Can you work these out from the model? Positions are in its coordinate system, mm. Face numbers are marked on the shaded views. A direction names the side the tool comes from. Coordinates: 2 decimals unless noted, no trailing zeros. Order: outer loops, then holes, each group sorted by start corner. A loop starts at its lowest first (then second) coordinate and runs counter-clockwise, first axis right, second up. Notation, with made-up numbers: M 15.25,40.5 L 38.25,40.5 A23 ccw 38.25,49.5 Z; hole C 70.5,29 d9. An arc over 180 degrees is marked long. Answer as CSV lines item,"result". Start each with the question number.
1. If we section it at A-A (x = 0): List the corners of the cut face in (y, z) for me.
2. If we mould it in two halves opening along Z, with no side actions, what happens to the marked faces 1, 2 and 3? For each: released by +Z, released by -Z, zero draft, split by the parting line, or undercut.
3. If we section it at C-C (z = -5): List the corners of the cut face in (x, y) for me.
4. If we section it at B-B (z = 0): List the corners of the cut face in (x, y) for me.
5. On a 3-axis mill with a long thin cutter (end or side, diameter ignored), from which of +Z, -Z, +X, -X, +Y, -Y can I reach the whole of each face in a straight line? I mean the marked faces 4, 5, 6 and 7. Say none if no direction works.
6. If we section it at D-D (x = 21): List the corners of the cut face in (y, z) for me, plus the area to 3 significant figures.
7. Will these pins go through, and if not, where does the flat tip stop? pin 1 (2 mm diameter, centred on y = 2.5, z = -11.5, fed in from +X); pin 2 (5 mm diameter, centred on y = 1, z = -11, fed in from -X); pin 3 (4.5 mm diameter, centred on x = -17, y = 4.5, fed in from +Z); pin 4 (2 mm diameter, centred on x = -21.92, z = 0, fed in from -Y).
8. I need wall thicknesses on line 1 along X through (y, z) = (7.9, 0); line 2 along X through (y, z) = (6, 0); line 3 along Z through (x, y) = (-22, 5). Which ranges of each line are inside material? Lowest first, please. Write a range as from..to.
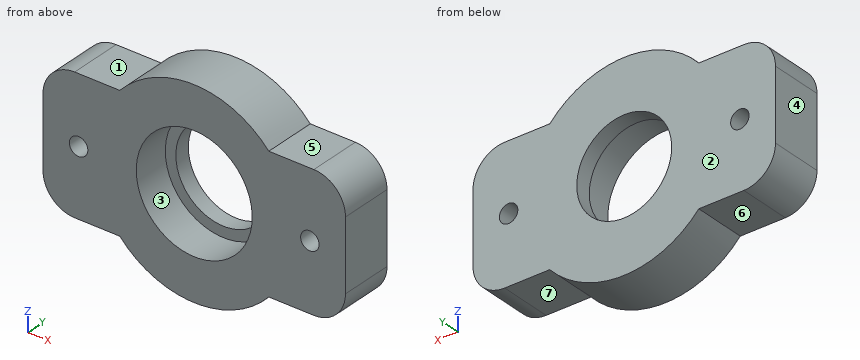
```python
from build123d import *

# Parameters (mm, degrees)
SKETCH1_R           = 11
SKETCH1_R_2         = 1.75
BOSS_EXTRUDE1_DEPTH = 10
BOSS_EXTRUDE2_START = -3
SKETCH2_R           = 11
SKETCH2_R_2         = 9
BOSS_EXTRUDE2_DEPTH = 3
FILLET1_R           = 6


with BuildPart() as part:
    # Sketch1 → Boss-Extrude1 (new body)
    with BuildSketch(Plane(origin=(0, 0, 0), x_dir=(1, 0, 0), z_dir=(0, 1, 0))):
        with BuildLine():
            Line((28.670310217, -12.7), (14.131878856, -12.7))
            ThreePointArc((14.131878856, -12.7), (0, -19), (-14.131878856, -12.7))
            Line((-14.131878856, -12.7), (-28.670310217, -12.7))
            Line((-28.670310217, -12.7), (-28.670310217, 12.7))
            Line((-28.670310217, 12.7), (-14.131878856, 12.7))
            ThreePointArc((-14.131878856, 12.7), (0, 19), (14.131878856, 12.7))
            Line((14.131878856, 12.7), (28.670310217, 12.7))
            Line((28.670310217, 12.7), (28.670310217, -12.7))
        make_face()
        with Locations(Location((0, 0, 0), (0, 0, 270))):
            Circle(SKETCH1_R, mode=Mode.SUBTRACT)
        with Locations(Location((21.920310217, 0, 0), (0, 0, 270))):
            Circle(SKETCH1_R_2, mode=Mode.SUBTRACT)
        with Locations(Location((-21.920310217, 0, 0), (0, 0, 270))):
            Circle(SKETCH1_R_2, mode=Mode.SUBTRACT)
    extrude(amount=BOSS_EXTRUDE1_DEPTH)

    # Sketch2 → Boss-Extrude2 (add)
    with BuildSketch(Plane(origin=(0, 10, 0), x_dir=(1, 0, 0), z_dir=(0, 1, 0)).offset(BOSS_EXTRUDE2_START)):
        with Locations(Location((0, 0, 0), (0, 0, 270))):
            Circle(SKETCH2_R)
        with Locations(Location((0, 0, 0), (0, 0, 270))):
            Circle(SKETCH2_R_2, mode=Mode.SUBTRACT)
    extrude(amount=BOSS_EXTRUDE2_DEPTH)

    # Fillet1
    fillet1_edges = [part.edges().sort_by_distance(p)[0] for p in [
        (28.670310217, 5, -12.7),
        (28.670310217, 5, 12.7),
        (-28.670310217, 5, 12.7),
        (-28.670310217, 5, -12.7),
    ]]
    fillet(fillet1_edges, radius=FILLET1_R)


solid = part.part
```
Solved:
1,outline,"M 0,-19 L 10,-19 L 10,-9 L 7,-9 L 7,-11 L 0,-11 Z; M 0,11 L 7,11 L 7,9 L 10,9 L 10,19 L 0,19 Z"
2,face 1,"released by +Z"
2,face 2,"zero draft"
2,face 3,"undercut"
3,outline,"M -28.67,0 L -9.8,0 L -9.8,7 L -7.48,7 L -7.48,10 L -28.67,10 Z; M 7.48,7 L 9.8,7 L 9.8,0 L 28.67,0 L 28.67,10 L 7.48,10 Z"
4,outline,"M -28.67,0 L -23.67,0 L -23.67,10 L -28.67,10 Z; M -20.17,0 L -11,0 L -11,7 L -9,7 L -9,10 L -20.17,10 Z; M 9,7 L 11,7 L 11,0 L 20.17,0 L 20.17,10 L 9,10 Z; M 23.67,0 L 28.67,0 L 28.67,10 L 23.67,10 Z"
5,face 4,"+Z, -Z, -X, +Y, -Y"
5,face 5,"+Z, +X, +Y, -Y"
5,face 6,"-Z, -X, +Y, -Y"
5,face 7,"-Z, +X, +Y, -Y"
6,outline,"M 0,-12.7 L 10,-12.7 L 10,-1.49 L 0,-1.49 Z; M 0,1.49 L 10,1.49 L 10,12.7 L 0,12.7 Z"
6,area,"224 mm²"
7,pin 1,"x = 27.31"
7,pin 2,"x = -28.39"
7,pin 3,"z = 12.7"
7,pin 4,"through"
8,line 1,"-28.67..-23.67, -20.17..-9, 9..20.17, 23.67..28.67"
8,line 2,"-28.67..-23.67, -20.17..-11, 11..20.17, 23.67..28.67"
8,line 3,"-12.7..-1.75, 1.75..12.7"
